Part model, mm, in its own coordinate system. A direction names the side the tool comes from. Round coordinates to 2 decimals unless told otherwise and drop trailing zeros. Loops run counter-clockwise (first coordinate to the right, second up) from the corner with the lowest first, then second, coordinate; pieces in that order, holes last. Notation, with made-up numbers: M 2.5,0 L 49.5,0 A20 ccw 49.5,30 Z; hole C 86.25,-14 d5. An arc over 180 degrees is marked long. Put each result on its own line as item: value. Start each with the question number.
1) Probe line 1 along X through (y, z) = (20, 57); line 2 along Z through (x, y) = (-5, -11); line 3 along X through (y, z) = (22, 73). List the from-to ranges inside material, lowest first.
2) Slice it at B-B on x = -6.5. Give the cut face in (y, z).
3) Which spindle directions (+Z, -Z, +X, -X, +Y, -Y) get a long thin tool onto all of the face, cutting with end or side? Do faces 1 (the flat face through (-1, -8, 19.05)), 2 (the flat face through (19.362, -17, 10)), 3 (the flat face through (-1, 0, 0)). Say none if no direction does.
4) Slice it at D-D on z = 27. Give the cut face in (x, y), then the cut area to 3 significant figures.
5) Slice it at A-A on y = 11. Give the cut face in (x, z), then the cut area to 3 significant figures.
6) Slice it at C-C on z = 70. Give the cut face in (x, y), then the cut area to 3 significant figures.
7) Drop flat-ended pins along their axis: pin 1 Ø8 at (x, y) = (-27.5, -20.5) entering from +Z; pin 2 Ø23 at (x, z) = (2, 75.5) entering from -Y; pin 3 Ø2 at (y, z) = (6.5, 77) entering from -X; pin 4 Ø9.5 at (x, z) = (32, 13.5) entering from -Y. Give the stop position or say it passes through.
8) Pull direction X, two halves, no side cores. Call faces 4 (the cylindrical face through (-27.552, 17.154, 83.793)), 5 (the flat face through (29, -7.53, 10)), 6 (the cylindrical face through (-4.068, 16.916, 37.402)): +X half, -X half, draft (parallel to the pull), parting line (faces both ways), or undercut.
```python
from build123d import *

# Parameters (mm, degrees)
F0_W     = 76.8338
F0_H     = 51.121704
F1_DEPTH = 19.05
F2_W     = 19.054732
F2_H     = 18.031149
F3_DEPTH = 22.606
F4_W     = 76.8338
F4_H     = 17.051882
F5_DEPTH = 76.2
F6_R     = 38.1
F7_R     = 20.228721
F8_DEPTH = 25.4


with BuildPart() as f1:
    # F0 (on Top) → F1 (new body)
    with BuildSketch(Plane.XY):
        Rectangle(F0_W, F0_H)
    extrude(amount=F1_DEPTH)

    # F2 (on face) → F3 (cut)
    with BuildSketch(Plane.XY.offset(19.05)):
        with Locations((28.889534, -16.545278)):
            Rectangle(F2_W, F2_H)
    extrude(amount=-F3_DEPTH, mode=Mode.SUBTRACT)

    # F4 (on face) → F5 (join)
    with BuildSketch(Plane.XY.offset(19.05)):
        with Locations((0, 17.034911)):
            Rectangle(F4_W, F4_H)
    extrude(amount=F5_DEPTH)

    # F6
    f6_edges = [f1.edges().sort_by_distance(p)[0] for p in [
        (-38.4169, 17.034911, 95.25),
        (38.4169, 17.034911, 95.25),
    ]]
    fillet(f6_edges, radius=F6_R)

    # F7 (on face) → F8 (cut)
    with BuildSketch(Plane.XZ.offset(-8.50897)):
        with Locations((0.3169, 57.15)):
            Circle(F7_R)
    extrude(amount=-F8_DEPTH, mode=Mode.SUBTRACT)


solid = f1.part
```
Recorded:
1. line 1: x = -38.42 to -19.91, 20.55 to 38.42
1. line 2: z = 0 to 19.05
1. line 3: x = -34.96 to -12.25, 12.89 to 34.96
2. outline: M -25.56,0 L 25.56,0 L 25.56,38.1 L 8.51,38.1 L 8.51,19.05 L -25.56,19.05 Z; M 8.51,76.2 L 25.56,76.2 L 25.56,94.74 L 8.51,94.74 Z
3. face 1: +Z, +X, -X, -Y
3. face 2: +Z, -Z, +X, -Y
3. face 3: -Z, +X, -X, +Y, -Y
4. outline: M -38.42,8.51 L 38.42,8.51 L 38.42,25.56 L -38.42,25.56 Z
4. area: 1,310 mm2
5. outline: M -38.42,0 L 38.42,0 L 38.42,57.15 A38.1 ccw 0.32,95.25 L -0.32,95.25 A38.1 ccw -38.42,57.15 Z; hole C 0.32,57.15 d40.46
5. area: 5,410 mm2
6. outline: M -36.18,8.51 L -15.31,8.51 L -15.31,25.56 L -36.18,25.56 Z; M 15.94,8.51 L 36.18,8.51 L 36.18,25.56 L 15.94,25.56 Z
6. area: 701 mm2
7. pin 1: stops at z = 19.05
7. pin 2: stops at y = 8.51
7. pin 3: passes through
7. pin 4: stops at y = -7.53
8. face 4: -X half
8. face 5: draft
8. face 6: undercut
